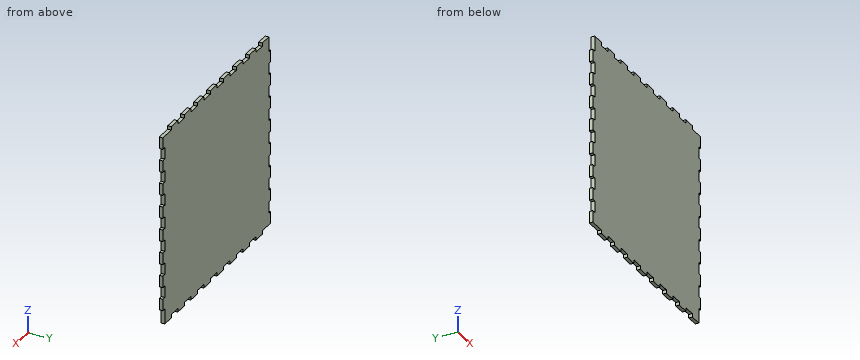
from build123d import *

# Parameters (mm, degrees)
BOSS_EXTRUDE1_DEPTH = 3


with BuildPart() as part:
    # Sketch1 → Boss-Extrude1 (new body)
    with BuildSketch(Plane(origin=(0, 0, 0), x_dir=(1, 0, 0), z_dir=(0, 1, 0))):
        Polygon((80, 80), (80, 70), (83, 70), (83, 60), (80, 60), (80, 50), (83, 50), (83, 40), (80, 40), (80, 30), (83, 30), (83, 20), (80, 20), (80, 10), (83, 10), (83, 0), (80, 0), (80, -10), (83, -10), (83, -20), (80, -20), (80, -30), (83, -30), (83, -40), (80, -40), (80, -50), (83, -50), (83, -60), (80, -60), (80, -70), (83, -70), (83, -80), (80, -80), (70, -80), (70, -83), (60, -83), (60, -80), (50, -80), (50, -83), (40, -83), (40, -80), (30, -80), (30, -83), (20, -83), (20, -80), (10, -80), (10, -83), (0, -83), (0, -80), (-10, -80), (-10, -83), (-20, -83), (-20, -80), (-30, -80), (-30, -83), (-40, -83), (-40, -80), (-50, -80), (-50, -83), (-60, -83), (-60, -80), (-70, -80), (-70, -83), (-80, -83), (-80, -80), (-80, -70), (-83, -70), (-83, -60), (-80, -60), (-80, -50), (-83, -50), (-83, -40), (-80, -40), (-80, -30), (-83, -30), (-83, -20), (-80, -20), (-80, -10), (-83, -10), (-83, 0), (-80, 0), (-80, 10), (-83, 10), (-83, 20), (-80, 20), (-80, 30), (-83, 30), (-83, 40), (-80, 40), (-80, 50), (-83, 50), (-83, 60), (-80, 60), (-80, 70), (-83, 70), (-83, 80), (-80, 80), (-70, 80), (-70, 83), (-60, 83), (-60, 80), (-50, 80), (-50, 83), (-40, 83), (-40, 80), (-30, 80), (-30, 83), (-20, 83), (-20, 80), (-10, 80), (-10, 83), (0, 83), (0, 80), (10, 80), (10, 83), (20, 83), (20, 80), (30, 80), (30, 83), (40, 83), (40, 80), (50, 80), (50, 83), (60, 83), (60, 80), (70, 80), (70, 83), (80, 83), align=None)
    extrude(amount=BOSS_EXTRUDE1_DEPTH)


solid = part.part
The model under review builds one solid part; all positions refer to its coordinate system, in mm. Give positions to 0.01 mm unless a question says otherwise; leave off trailing zeros. Order: outer loops, then holes, each group sorted by start corner. A loop starts at its lowest first (then second) coordinate and runs counter-clockwise, first axis right, second up. Notation, with made-up numbers: M 21.5,15 L 61.5,15 A29 cw 61.5,44 Z; hole C 35.5,1.25 d1. An arc over 180 degrees is marked long. One line per question, with ' | ' between items. Start each with the question number.
1) Consider section A-A, the plane z = -18. Give the boundary of the cut face in (x, y).
2) Consider section B-B, the plane x = 45.5. Give the boundary of the cut face in (y, z).
3) Wall thickness on L1, parallel to X at y = 1.85, z = -30.5; L2, parallel to Z at x = 40.5, y = 1.3: over which ranges is each line inside the solid? List them lowest first. Write a range as from..to.
4) Clearance check with flat-ended pins moving along their axes: P1, Ø0.9, axis at y = 2, z = -43, coming from the -X side; P2, Ø0.9, axis at y = 2, z = -81.5, coming from the -X side; P3, Ø1, axis at y = 2, z = 21, coming from the +X side. State where each tip first meets the part, or that it passes through.
Found:
1) outline: M -83,0 L 80,0 L 80,3 L -83,3 Z
2) outline: M 0,-80 L 3,-80 L 3,83 L 0,83 Z
3) L1: x = -83..80 | L2: z = -80..83
4) P1: stops at x = -80 | P2: stops at x = -70 | P3: stops at x = 80
